The model under review builds one solid part; all positions refer to its coordinate system, in mm. Face numbers are marked on the shaded views. A direction names the side the tool comes from. Round coordinates to 2 decimals unless told otherwise and drop trailing zeros. Order: outer loops, then holes, each group sorted by start corner. A loop starts at its lowest first (then second) coordinate and runs counter-clockwise, first axis right, second up.
1) Clearance check with flat-ended pins moving along their axes: P1, Ø4, axis at x = -2.5, z = 0.5, coming from the +Y side; P2, Ø1.5, axis at x = -0.5, y = 1.5, coming from the -Z side; P3, Ø3, axis at x = -2.5, z = 1, coming from the -Y side. State where each tip first meets the part, or that it passes through.
2) To check wall thickness, follow L1, parallel to Y at x = 0, z = -5; L2, parallel to X at y = 2, z = 8.5; L3, parallel to Z at x = -2, y = -0.75. State the ranges of each line that lie inside material, in increasing order.
3) Machinability: for the marked faces 1 and 2, which of the approach directions +Z, -Z, +X, -X, +Y, -Y give a long, thin tool a straight path to every point of the face, cutting with its end or side? Answer none if there is none.
4) Mouldability with a two-part tool opening along Y and no side actions: class the marked faces 3, 4 and 5 as pulls with the +Y half, pulls with the -Y half, needs draft (parallel to the pull), parting line crosses it, or undercut.
5) Consider section C-C (y = -1.5). Give the boundary of the cut face in (x, z) (3 decimals).
6) Consider section A-A (z = -1.75). Give the boundary of the cut face in (x, y) (1 decimal).
7) Consider section D-D (z = 0.75). Give the boundary of the cut face in (x, y) (1 decimal).
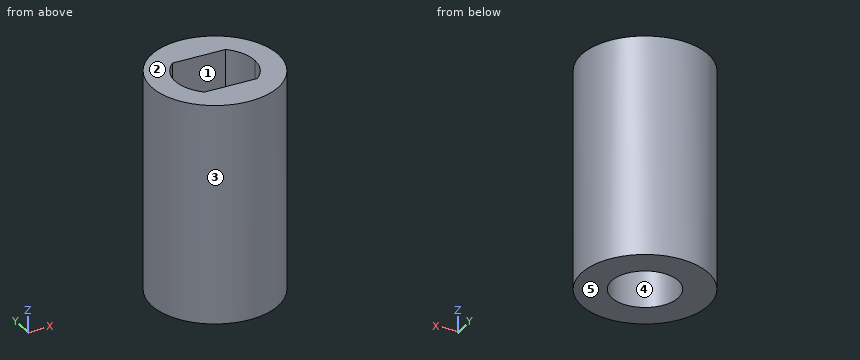
from build123d import *

# Parameters (mm, degrees)
F0_R          = 4.7625
F1_DEPTH      = 9.525
F1_DEPTH_BACK = 7
F4_DEPTH      = 9.526
F3_R          = 2.5
F5_DEPTH      = 7.001
F6_DEPTH      = 1.27


with BuildPart() as f1:
    # F0 (on Top) → F1 (new body, two sides)
    with BuildSketch(Plane.XY) as f1_sk:
        Circle(F0_R)
    extrude(amount=F1_DEPTH)
    extrude(f1_sk.sketch, amount=-F1_DEPTH_BACK)

    # F2 (on Top) → F4 (cut, through all)
    with BuildSketch(Plane.XY):
        with BuildLine():
            ThreePointArc((1.984313, -2.25), (2.734313, -1.234313), (3, 0))
            ThreePointArc((3, 0), (2.734313, 1.234313), (1.984313, 2.25))
            Line((1.984313, 2.25), (-1.984313, 2.25))
            ThreePointArc((-1.984313, 2.25), (-3, 0), (-1.984313, -2.25))
            Line((-1.984313, -2.25), (1.984313, -2.25))
        make_face()
    extrude(amount=F4_DEPTH, mode=Mode.SUBTRACT)

    # F3 (on Top) → F5 (cut, through all)
    with BuildSketch(Plane.XY):
        Circle(F3_R)
    extrude(amount=-F5_DEPTH, mode=Mode.SUBTRACT)

    # F0 (on Top) → F6 (join)
    with BuildSketch(Plane.XY):
        Circle(F0_R)
    extrude(amount=F6_DEPTH)


solid = f1.part
Answer below:
1. P1: stops at y = 4.74
1. P2: stops at z = 0
1. P3: stops at y = -4.66
2. L1: y = -4.76 to -2.5, 2.5 to 4.76
2. L2: x = -4.32 to -2.24, 2.24 to 4.32
2. L3: z = 0 to 1.27
3. face 1: +Z
3. face 2: +Z, +X, -X, +Y, -Y
4. face 3: parting line crosses it
4. face 4: undercut
4. face 5: needs draft
5. outline: (-4.52, -7) - (-2, -7) - (-2, 0) - (2, 0) - (2, -7) - (4.52, -7) - (4.52, 9.525) - (2.598, 9.525) - (2.598, 1.27) - (-2.598, 1.27) - (-2.598, 9.525) - (-4.52, 9.525) - close
6. outline: circle Ø9.5 at (0, 0); hole circle Ø5 at (0, 0)
7. outline: circle Ø9.5 at (0, 0)
